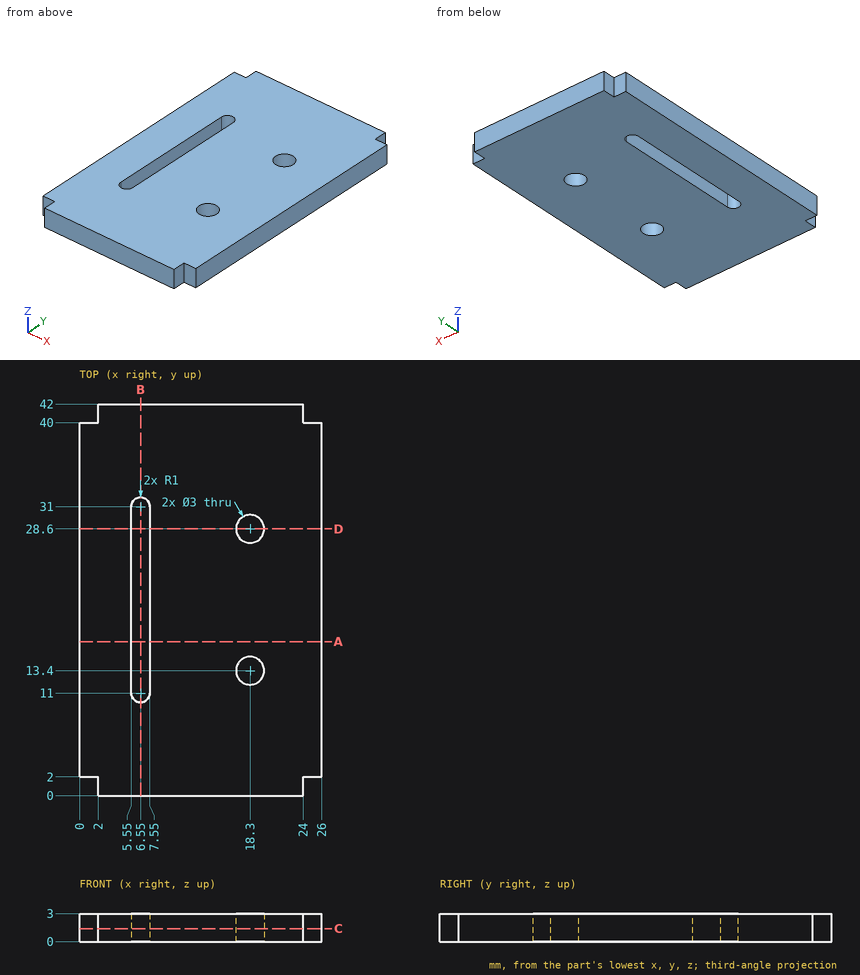
Input: dimensioned drawing with shaded views. Units: mm. Origin: part minimum x, y, z. Coordinates: 2 decimals unless noted, no trailing zeros. Loops run counter-clockwise (first coordinate to the right, second up) from the corner with the lowest first, then second, coordinate; pieces in that order, holes last.
Q1. Section B-B, the plane x = 6.55. Return the cut outline in (y, z).
Results are:
outline: (0, 0) - (10, 0) - (10, 3) - (0, 3) - close; (32, 0) - (42, 0) - (42, 3) - (32, 3) - close
Q2. Section A-A, the plane y = 16.5. Return the cut outline in (x, z), and give its area (3 significant figures).
Results are:
outline: (0, 0) - (5.55, 0) - (5.55, 3) - (0, 3) - close; (7.55, 0) - (26, 0) - (26, 3) - (7.55, 3) - close
area: 72.0 mm2
Q3. Section D-D, the plane y = 28.6. Return the cut outline in (x, z), and give its area (3 significant figures).
Results are:
outline: (0, 0) - (5.55, 0) - (5.55, 3) - (0, 3) - close; (7.55, 0) - (16.8, 0) - (16.8, 3) - (7.55, 3) - close; (19.8, 0) - (26, 0) - (26, 3) - (19.8, 3) - close
area: 63.0 mm2
Q4. Contact query for flat-ended pins moving along their axis: pin 1 (1.6 mm diameter, centred on x = 25, z = 2, fed in from +Y); pin 2 (5 mm diameter, centred on x = 18.3, y = 13.4, fed in from -Z); pin 3 (1.6 mm diameter, centred on x = 0.5, z = 2, fed in from -Y); pin 4 (1 mm diameter, centred on y = 41.5, z = 1, fed in from -X). Output: stop coordinate, or through.
Results are:
pin 1: stops at y = 40
pin 2: stops at z = 0
pin 3: stops at y = 2
pin 4: stops at x = 2
Q5. Section C-C, the plane z = 1.4. Return the cut outline in (x, y).
Results are:
outline: (0, 2) - (2, 2) - (2, 0) - (24, 0) - (24, 2) - (26, 2) - (26, 40) - (24, 40) - (24, 42) - (2, 42) - (2, 40) - (0, 40) - close; hole (5.55, 11) arc R1 ccw to (7.55, 11) - (7.55, 31) arc R1 ccw to (5.55, 31) - close; hole circle Ø3 at (18.3, 13.4); hole circle Ø3 at (18.3, 28.6)
Q6. Line query: line 1 along Y through (x, z) = (18.3, 1.15); line 2 along X through (y, z) = (21.5, 2.45); line 3 along Y through (x, z) = (24.5, 1.1). Output: solid intervals per line, ascending.
Results are:
line 1: y = 0 to 11.9, 14.9 to 27.1, 30.1 to 42
line 2: x = 0 to 5.55, 7.55 to 26
line 3: y = 2 to 40
